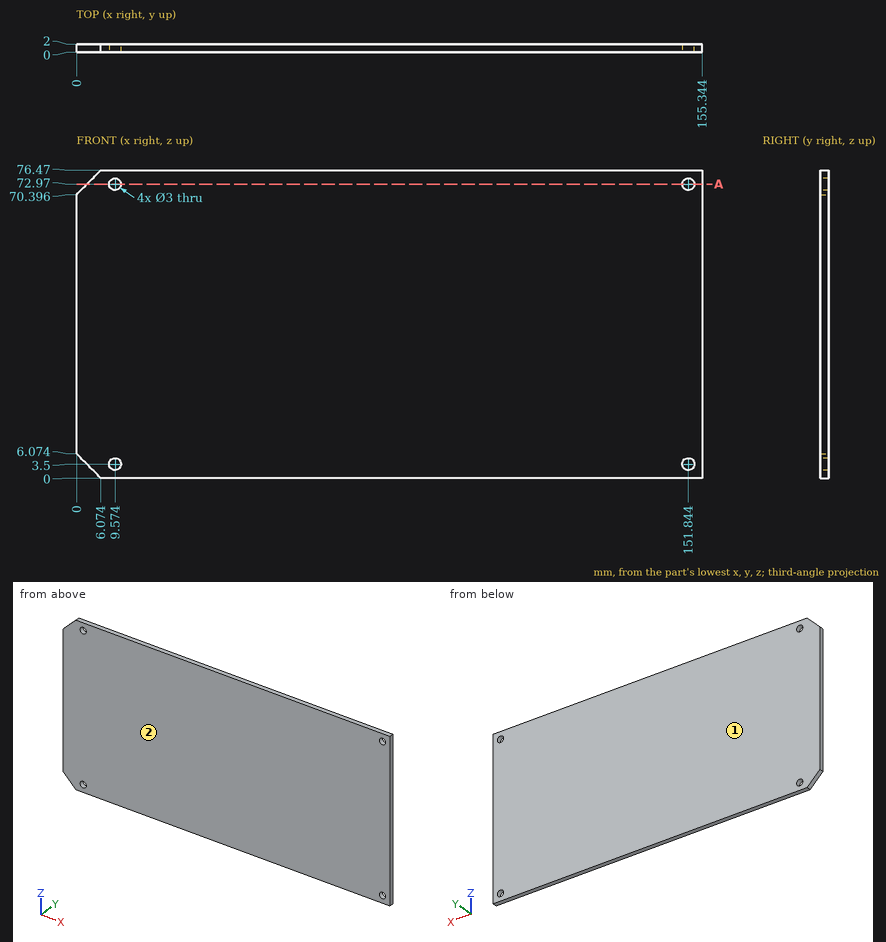
Print and shaded views of the part. All mm, measured from the part's lowest x, y and z. Coordinates: 2 decimals unless noted, no trailing zeros. Order: outer loops, then holes, each group sorted by start corner. A loop starts at its lowest first (then second) coordinate and runs counter-clockwise, first axis right, second up.
Item 1: Drill centre lines: L1, parallel to X at y = 0.9, z = 72.97; L2, parallel to X at y = 0.5, z = 3; L3, parallel to Z at x = 9, y = 1.95. Where is each one in solid material? Low to high.
Filled in:
L1: x = 2.57 to 8.07, 11.07 to 150.34, 153.34 to 155.34
L2: x = 3.07 to 8.16, 10.99 to 150.43, 153.26 to 155.34
L3: z = 0 to 2.11, 4.89 to 71.58, 74.36 to 76.47
Item 2: Mould opens along Y. For the marked faces 1 and 2 say: released by +Y, released by -Y, zero draft, split by the parting line, or undercut.
Filled in:
face 1: released by +Y
face 2: released by -Y
Item 3: Drop a flat-ended pin along its axis: pin 1 Ø2.5 at (x, z) = (151.84, 3.5) entering from +Y. Give the stop position or say it passes through.
Filled in:
pin 1: passes through
Item 4: Saw through at A-A on z = 72.97. List the corners of the cut face in (x, y).
Filled in:
outline: (2.57, 0) - (8.07, 0) - (8.07, 2) - (2.57, 2) - close; (11.07, 0) - (150.34, 0) - (150.34, 2) - (11.07, 2) - close; (153.34, 0) - (155.34, 0) - (155.34, 2) - (153.34, 2) - close
